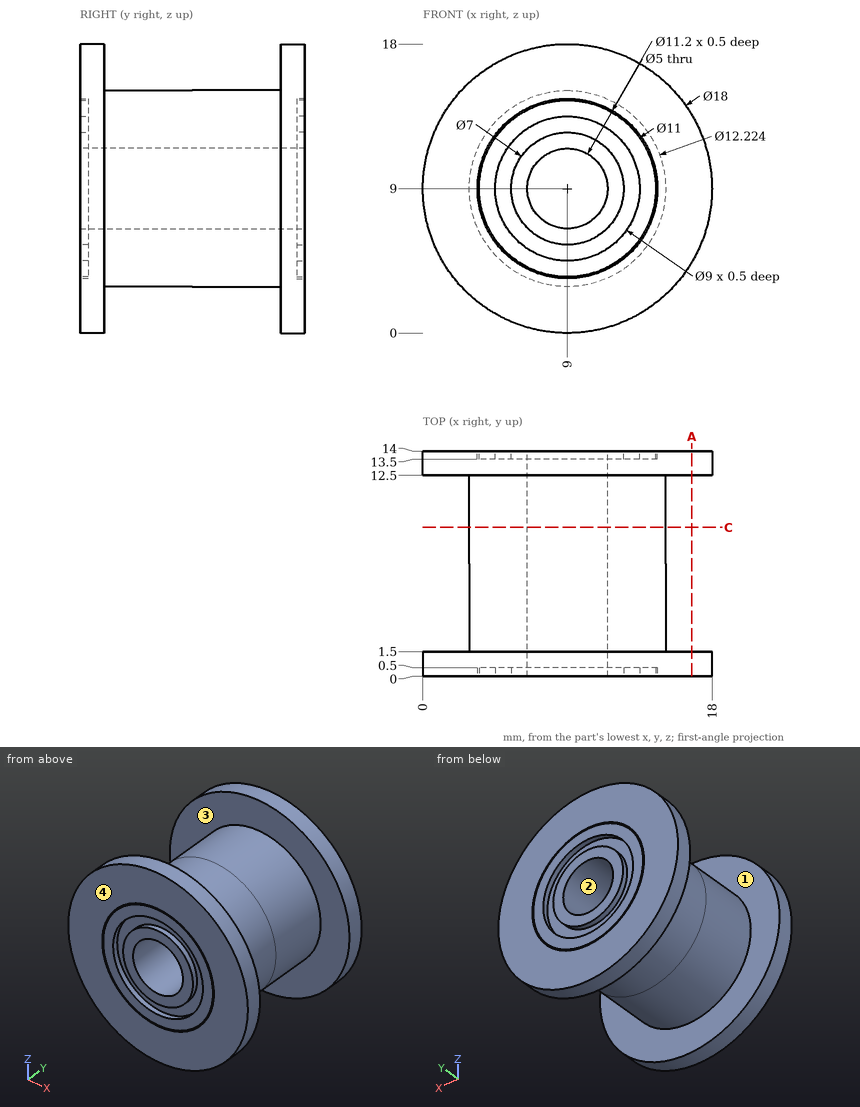
Design review of the part shown in the three views and the two pictorial views. Dimensions are in mm from the part's minimum x, y and z. A direction names the side the tool comes from. Give positions to 0.01 mm unless a question says otherwise; leave off trailing zeros. Order: outer loops, then holes, each group sorted by start corner. A loop starts at its lowest first (then second) coordinate and runs counter-clockwise, first axis right, second up. Notation, with made-up numbers: M 41,-12 L 82,-12 A31 ccw 82,24 Z; hole C -25,85.25 d6. An arc over 180 degrees is marked long. Answer in a Markdown table with one row per item. Add a question column.
(1) Consider section C-C on y = 9.25. State the section outline as (x, z) points (1 decimal).
(2) For pin 1 (2.5 mm diameter, centred on x = 10, z = 9.5, fed in from -Y); pin 2 (2 mm diameter, centred on y = 12, z = 11, fed in from -X); pin 3 (8 mm diameter, centred on x = 6, y = 6, fed in from -Z); pin 4 (5 mm diameter, centred on y = 7, z = 15.5, fed in from +X), all flat-tipped, find the tip position at first contact; note any pin that passes through.
(3) For the marked faces 3 and 4, list the 3-axis set-ups (+Z, -Z, +X, -X, +Y, -Y) from which the entire face can be reached by the end or side of a thin tool; tool diameter is ignored.
(4) Wall thickness on probe 1 along Y at (x, z) = (3.25, 6); probe 2 along X at (y, z) = (4, 7.25) (1 decimal); probe 3 along Z at (x, y) = (8, 4.25): over which ranges is each line inside the solid? List them lowest first. Write a range as [from, to].
(5) Consider section A-A on x = 16.75. State the section outline as (y, z) points (1 decimal).
(6) Mouldability with a two-part tool opening along Z and no side actions: class the marked faces 1 and 2 as +Z half, -Z half, draft (parallel to the pull), parting line (faces both ways), or undercut.
Evaluation:
| question | item | result |
|---|---|---|
| 1 | outline | C 9,9 d12.2; hole C 9,9 d5 |
| 2 | pin 1 | passes through |
| 2 | pin 2 | stops at x = 0.07 |
| 2 | pin 3 | stops at z = 2.89 |
| 2 | pin 4 | stops at x = 13.62 |
| 3 | face 3 | none |
| 3 | face 4 | +Z, -Z, +X, -X, -Y |
| 4 | probe 1 | y = [0, 1.5], [12.5, 14] |
| 4 | probe 2 | x = [3.1, 7.2], [10.8, 14.9] |
| 4 | probe 3 | z = [2.97, 6.71], [11.29, 15.03] |
| 5 | outline | M 0,4.4 L 1.5,4.4 L 1.5,13.6 L 0,13.6 Z; M 12.5,4.4 L 14,4.4 L 14,13.6 L 12.5,13.6 Z |
| 6 | face 1 | draft |
| 6 | face 2 | undercut |
